The model under review builds one solid part; all positions refer to its coordinate system, in mm. A direction names the side the tool comes from. Round coordinates to 2 decimals unless told otherwise and drop trailing zeros. Loops run counter-clockwise (first coordinate to the right, second up) from the corner with the lowest first, then second, coordinate; pieces in that order, holes last. Notation, with made-up numbers: (79, -31.75) -> (91, -31.75) arc R27 cw to (91, -5.75) -> close; hole circle Ø10 at (-31, -20.5). An arc over 180 degrees is marked (long way). Use a Markdown table: item, result. Add a question column.
1) For faces 4 (the flat face through (0, 7.85, -291.18)), 5 (the cylindrical face through (1.97, -5.17, -292.47)), list the 3-axis set-ups (+Z, -Z, +X, -X, +Y, -Y) from which the entire face can be reached by the end or side of a thin tool; tool diameter is ignored.
2) Wall thickness on probe 1 along Y at (x, z) = (3.1, -41); probe 2 along Z at (x, y) = (-5.25, 1); probe 3 along Y at (x, z) = (2.3, -83): over which ranges is each line inside the solid? List them lowest first.
3) Insertion check: pin 1 (1.5 mm diameter, centred on y = 4, z = -267, fed in from -X); pin 2 (6 mm diameter, centred on x = -0.5, z = -190.5, fed in from +Y); pin 3 (2 mm diameter, centred on x = -3.5, y = -18, fed in from +Z); pin 4 (0.9 mm diameter, centred on y = 16.5, z = -280.5, fed in from -X). Each pin has a flat end and moves straight along its axis. Give the tip position at first contact, or say it passes through.
4) Consider section A-A on x = -4.25. Give the boundary of the cut face in (y, z).
5) Mouldability with a two-part tool opening along Z and no side actions: class faces 1 (the cylindrical face through (1.972, -1.275, 57.986)), 2 (the cylindrical face through (-3.549, -5.745, -266.144)), 3 (the flat face through (4, 1, -143)) as released by +Z, released by -Z, zero draft, split by the parting line, or undercut.
6) Consider section B-B on z = -192. Give the boundary of the cut face in (x, y), plus the area to 3 significant figures.
from build123d import *

# Parameters (mm, degrees)
SKETCH1_R           = 28
SKETCH1_R_2         = 13.5
BOSS_EXTRUDE1_DEPTH = 4
SKETCH2_R           = 34
SKETCH2_R_2         = 29
SKETCH2_R_3         = 20
SKETCH2_R_4         = 15
BOSS_EXTRUDE2_DEPTH = 7
CHAMFER1_SIZE       = 8
SKETCH3_R           = 2
CUT_EXTRUDE1_DEPTH  = 344.011661609
SKETCH4_R           = 1.5
CUT_EXTRUDE2_DEPTH  = 344.116598258
SKETCH5_R           = 1.5
CUT_EXTRUDE3_DEPTH  = 5


with BuildPart() as part:
    # Sketch1 → Boss-Extrude1 (new body)
    with BuildSketch(Plane(origin=(0, 0, 0), x_dir=(0, 0, -1), z_dir=(1, 0, 0))):
        with BuildLine():
            Line((0, 58), (280, 58))
            ThreePointArc((280, 58), (338, 0), (280, -58))
            Line((280, -58), (0, -58))
            ThreePointArc((0, -58), (-58, 0), (0, 58))
        make_face()
        Circle(SKETCH1_R, mode=Mode.SUBTRACT)
        with Locations((280, 0)):
            Circle(SKETCH1_R_2, mode=Mode.SUBTRACT)
    extrude(amount=BOSS_EXTRUDE1_DEPTH)

    # Sketch2 → Boss-Extrude2 (add)
    # profile 1 of 2: a face of its own
    with BuildSketch(Plane.ZY.offset(7)):
        Circle(SKETCH2_R)
        Circle(SKETCH2_R_2, mode=Mode.SUBTRACT)
    # profile 2 of 2: a face of its own
    with BuildSketch(Plane.ZY.offset(7)):
        with Locations((-280, 0)):
            Circle(SKETCH2_R_3)
        with Locations((-280, 0)):
            Circle(SKETCH2_R_4, mode=Mode.SUBTRACT)
    extrude(amount=-BOSS_EXTRUDE2_DEPTH)

    # Chamfer1
    # the kernel refuses this chamfer: 8 mm, written as the material it adds along each edge
    with BuildSketch(Plane(origin=(0, 0, 0), x_dir=(0, 0, 1), z_dir=(0, -1, 0))) as chamfer1_piece_1_section:
        Polygon((34 + CHAMFER1_SIZE, 0), (34, CHAMFER1_SIZE), (34, 0), align=None)
    chamfer1_piece_1 = revolve(axis=Axis((0, 0, 0), (-1, 0, 0)), mode=Mode.PRIVATE)
    chamfer1_piece_1 = split(chamfer1_piece_1, bisect_by=Plane(origin=(-7, 0, -38.472213865), z_dir=(1, 0, 0)), keep=Keep.TOP, mode=Mode.PRIVATE)
    add(chamfer1_piece_1)
    with BuildSketch(Plane(origin=(0, 0, -280), x_dir=(0, 0, 1), z_dir=(0, -1, 0))) as chamfer1_piece_2_section:
        Polygon((20 + CHAMFER1_SIZE, 0), (20, CHAMFER1_SIZE), (20, 0), align=None)
    chamfer1_piece_2 = revolve(axis=Axis((0, 0, -280), (-1, 0, 0)), mode=Mode.PRIVATE)
    chamfer1_piece_2 = split(chamfer1_piece_2, bisect_by=Plane(origin=(-7, 0, -304.493064149), z_dir=(1, 0, 0)), keep=Keep.TOP, mode=Mode.PRIVATE)
    add(chamfer1_piece_2)

    # Sketch3 → Cut-Extrude1 (cut, through all)
    with BuildSketch(Plane.ZY):
        with Locations((-66, 50)):
            Circle(SKETCH3_R)
        with Locations(Location((-66, -50, 0), (0, 0, 180))):
            Circle(SKETCH3_R)
        with Locations((-83, -50)):
            Circle(SKETCH3_R)
        with Locations(Location((-83, 50, 0), (0, 0, 180))):
            Circle(SKETCH3_R)
    extrude(amount=-CUT_EXTRUDE1_DEPTH, mode=Mode.SUBTRACT)

    # Sketch4 → Cut-Extrude2 (cut, through all)
    with BuildSketch(Plane(origin=(4, 0, 0), x_dir=(0, 0, -1), z_dir=(1, 0, 0))):
        with Locations((-29.5, 42)):
            Circle(SKETCH4_R)
        with Locations((41, 54)):
            Circle(SKETCH4_R)
        with Locations((41, 31)):
            Circle(SKETCH4_R)
    extrude(amount=-CUT_EXTRUDE2_DEPTH, mode=Mode.SUBTRACT)

    # Sketch5 → Cut-Extrude3 (cut)
    with BuildSketch(Plane.ZY.offset(7)):
        with Locations((-280, 17)):
            Circle(SKETCH5_R)
        with Locations((-263, 0)):
            Circle(SKETCH5_R)
        with Locations((-280, -17)):
            Circle(SKETCH5_R)
        with Locations((-297, 0)):
            Circle(SKETCH5_R)
    extrude(amount=-CUT_EXTRUDE3_DEPTH, mode=Mode.SUBTRACT)


solid = part.part
Result set:
| question | item | result |
|---|---|---|
| 1 | face 4 | -X |
| 1 | face 5 | +X, -X |
| 2 | probe 1 | -58 to 29.5, 32.5 to 52.5, 55.5 to 58 |
| 2 | probe 2 | -302.73 to -298.12, -295.88 to -294.97, -265.03 to -264.12, -261.88 to -257.27, -36.74 to -28.98, 28.98 to 36.74 |
| 2 | probe 3 | -58 to -52, -48 to 48, 52 to 58 |
| 3 | pin 1 | x = 0 |
| 3 | pin 2 | y = 58 |
| 3 | pin 3 | z = 35.27 |
| 3 | pin 4 | x = -2 |
| 4 | outline | circle Ø75.5 at (0, 0); circle Ø47.5 at (0, -280); hole circle Ø58 at (0, 0); hole circle Ø3 at (-17, -280); hole circle Ø30 at (0, -280); hole circle Ø3 at (0, -297); hole circle Ø3 at (0, -263); hole circle Ø3 at (17, -280) |
| 5 | face 1 | released by +Z |
| 5 | face 2 | undercut |
| 5 | face 3 | zero draft |
| 6 | outline | (0, -58) -> (4, -58) -> (4, 58) -> (0, 58) -> close |
| 6 | area | 464 mm2 |
